Part model, mm, in its own coordinate system. A direction names the side the tool comes from. Round coordinates to 2 decimals unless told otherwise and drop trailing zeros. Loops run counter-clockwise (first coordinate to the right, second up) from the corner with the lowest first, then second, coordinate; pieces in that order, holes last.
1) Band-saw the part on D-D, the plane y = -1.75. Write the cut outline in (x, z), then the cut area to 3 significant figures.
2) Band-saw the part on C-C, the plane z = 50. Write the cut outline in (x, y).
3) Band-saw the part on A-A, the plane y = -17. Write the cut outline in (x, z), then the cut area to 3 significant figures.
4) 3-axis set-ups, long thin cutter, end or side, ignore diameter. For faces 1 (the flat face through (-30.447, -23, 14)), 2 (the flat face through (-39, -13, -30.344)), 3 (the flat face through (-38, -21.59, 21)): which of +Z, -Z, +X, -X, +Y, -Y reach the whole face in a straight line?
5) Band-saw the part on B-B, the plane x = -28.75. Write the cut outline in (y, z), then the cut area to 3 significant figures.
6) Drop flat-ended pins along their axis: P1, Ø4, axis at y = -24, z = 5.5, coming from the -X side; P2, Ø6, axis at y = -22, z = 47, coming from the -X side; P3, Ø2, axis at x = -47, y = -17, coming from the +Z side. Give the stop position or say it passes through.
7) Probe line 1 (Y direction, x = -27.75, z = 32); line 2 (Z direction, x = -35.75, y = -6.25); line 3 (X direction, y = -24.5, z = 47.5). List the from-to ranges inside material, lowest first.
8) Mould opens along Y. For faces 4 (the flat face through (-29, -13, 76.336)), 5 (the flat face through (-29, -13, 72.526)), 6 (the flat face through (-38.5, 0, 17.3)) say: +Y half, -Y half, draft (parallel to the pull), parting line (faces both ways), or undercut.
from build123d import *

# Parameters (mm, degrees)
F1_DEPTH = 25.4
F2_W     = 17.78
F2_H     = 102.87
F3_DEPTH = 50.8


with BuildPart() as f1:
    # F0 (on Front) → F1 (new body)
    with BuildSketch(Plane.XZ):
        Polygon((-26.637435, 76.336338), (-30.447435, 76.336338), (-52.037435, -34.153662), (-26.637435, -34.153662), align=None)
        Polygon((-47.410897, -30.343662), (-30.447435, 56.469348), (-30.447435, -30.343662), align=None, mode=Mode.SUBTRACT)
    extrude(amount=F1_DEPTH)

    # F2 (on face) → F3 (cut)
    with BuildSketch(Plane.YZ.offset(-26.637435)):
        with Locations((-12.7, 21.091338)):
            Rectangle(F2_W, F2_H)
    extrude(amount=-F3_DEPTH, mode=Mode.SUBTRACT)


solid = f1.part
Reported:
1. outline: (-52.04, -34.15) - (-26.64, -34.15) - (-26.64, 76.34) - (-30.45, 76.34) - close; hole (-47.41, -30.34) - (-30.45, -30.34) - (-30.45, 56.47) - close
1. area: 877 mm2
2. outline: (-35.59, -25.4) - (-31.71, -25.4) - (-31.71, -21.59) - (-35.59, -21.59) - close; (-35.59, -3.81) - (-31.71, -3.81) - (-31.71, 0) - (-35.59, 0) - close; (-30.45, -25.4) - (-26.64, -25.4) - (-26.64, -21.59) - (-30.45, -21.59) - close; (-30.45, -3.81) - (-26.64, -3.81) - (-26.64, 0) - (-30.45, 0) - close
3. outline: (-52.04, -34.15) - (-26.64, -34.15) - (-26.64, -30.34) - (-51.29, -30.34) - close; (-31.19, 72.53) - (-26.64, 72.53) - (-26.64, 76.34) - (-30.45, 76.34) - close
3. area: 111 mm2
4. face 1: +Y, -Y
4. face 2: none
4. face 3: +X, -X
5. outline: (-25.4, -34.15) - (0, -34.15) - (0, 76.34) - (-25.4, 76.34) - close; hole (-21.59, -30.34) - (-3.81, -30.34) - (-3.81, 72.53) - (-21.59, 72.53) - close
5. area: 977 mm2
6. P1: stops at x = -44.68
6. P2: stops at x = -36.77
6. P3: stops at z = -30.34
7. line 1: y = -25.4 to -21.59, -3.81 to 0
7. line 2: z = -34.15 to -30.34
7. line 3: x = -36.08 to -32.2, -30.45 to -26.64
8. face 4: draft
8. face 5: undercut
8. face 6: +Y half
